from build123d import *

# Parameters (mm, degrees)
F0_W           = 70
F0_H           = 50
F1_DEPTH       = 850
F3_D           = 8
F3_DEPTH       = 22
F3_TIP         = 2.4034424761
F5_D           = 8.2
F5_CSINK_D     = 17.3
F5_CSINK_ANGLE = 90


with BuildPart() as f1:
    # F0 (on Top) → F1 (new body)
    with BuildSketch(Plane.XY):
        Rectangle(F0_W, F0_H)
    extrude(amount=F1_DEPTH)

    # F3
    with Locations(Plane.YZ.offset(35)):
        with Locations((0, 215), (0, 255), (0, 795), (0, 835)):
            Hole(F3_D / 2, depth=F3_DEPTH)
            with Locations((0, 0, -(F3_DEPTH + F3_TIP / 2))):  # 118° drill point
                Cone(0, F3_D / 2, F3_TIP, mode=Mode.SUBTRACT)

    # F5 (through all)
    with Locations(Plane.XZ.offset(25)):
        with Locations((-10, 235), (-10, 815)):
            CounterSinkHole(F5_D / 2, F5_CSINK_D / 2, counter_sink_angle=F5_CSINK_ANGLE)


solid = f1.part
Verification items for the finished model (mm, model axes). Coordinates: 2 decimals unless noted, no trailing zeros. Put each result on its own line as item: value. Start each with the question number.
1. Go/stop test with flat-tipped pins: pin 1 Ø13 at (x, z) = (-10, 235) entering from -Y; pin 2 Ø6.5 at (y, z) = (0, 255) entering from +X. Record where each tip stops, or that it passes through.
2. Material ranges on L1, parallel to Z at x = 18, y = 0; L2, parallel to Y at x = 20, z = 795; L3, parallel to Z at x = -8.5, y = -4, recorded low to high. Write a range as [from, to].
3. Mould release check, pull along X, two halves, no side actions. Record for faces 1 (the flat face through (35, 0, 419)), 2 (the flat face through (0, 0, 850)), 3 (the conical face through (-9.063, -20.671, 810.782)): released by +X, released by -X, zero draft, split by the parting line, or undercut.
Computed:
1. pin 1: y = -22.85
1. pin 2: x = 12.55
2. L1: [0, 211], [219, 251], [259, 791], [799, 831], [839, 850]
2. L2: [-25, -4], [4, 25]
2. L3: [0, 231.18], [238.82, 811.18], [818.82, 850]
3. face 1: released by +X
3. face 2: zero draft
3. face 3: undercut
